Can you work these out from the model? Positions are in its coordinate system, mm. Face numbers are marked on the shaded views. A direction names the side the tool comes from. Round coordinates to 2 decimals unless told otherwise and drop trailing zeros. Loops run counter-clockwise (first coordinate to the right, second up) from the corner with the lowest first, then second, coordinate; pieces in that order, holes last. Notation, with made-up numbers: M 52.25,-30 L 65.25,-30 A38 ccw 65.25,8 Z; hole C 67,17 d7. An arc over 180 degrees is marked long. Return JSON: item names as keys, results as strings.
```python
from build123d import *

# Parameters (mm, degrees)
SKETCH1_W           = 40
SKETCH1_H           = 40
BOSS_EXTRUDE1_DEPTH = 12.7
SKETCH2_R           = 2.67558437
CUT_EXTRUDE1_DEPTH  = 8
CUT_EXTRUDE1_TAPER  = 17.5
FILLET1_R           = 3.175
SKETCH3_W           = 7.62
SKETCH3_H           = 1.27
BOSS_EXTRUDE2_DEPTH = 7.62
SKETCH4_W           = 1.27
SKETCH4_H           = 7.62
BOSS_EXTRUDE3_DEPTH = 7.62
SKETCH5_W           = 1.27
SKETCH5_H           = 7.62
BOSS_EXTRUDE4_DEPTH = 7.62
SKETCH6_W           = 7.62
SKETCH6_H           = 1.27
BOSS_EXTRUDE5_DEPTH = 7.62
SKETCH7_R           = 1.6256
CUT_EXTRUDE2_DEPTH  = 7.62


with BuildPart() as part:
    # Sketch1 → Boss-Extrude1 (new body)
    with BuildSketch(Plane.XY):
        with Locations((-32.473746891, -5.437780853)):
            Rectangle(SKETCH1_W, SKETCH1_H)
    extrude(amount=BOSS_EXTRUDE1_DEPTH)

    # Sketch2 → Cut-Extrude1 (cut)
    with BuildSketch(Plane.XY.offset(12.7)):
        with Locations((-45.973746891, 8.062219147)):
            Circle(SKETCH2_R)
        with Locations((-36.973746891, 8.062219147)):
            Circle(SKETCH2_R)
        with Locations((-27.973746891, 8.062219147)):
            Circle(SKETCH2_R)
        with Locations((-18.973746891, 8.062219147)):
            Circle(SKETCH2_R)
        with Locations((-45.973746891, -0.937780853)):
            Circle(SKETCH2_R)
        with Locations((-36.973746891, -0.937780853)):
            Circle(SKETCH2_R)
        with Locations((-27.973746891, -0.937780853)):
            Circle(SKETCH2_R)
        with Locations((-18.973746891, -0.937780853)):
            Circle(SKETCH2_R)
        with Locations((-45.973746891, -9.937780853)):
            Circle(SKETCH2_R)
        with Locations((-36.973746891, -9.937780853)):
            Circle(SKETCH2_R)
        with Locations((-27.973746891, -9.937780853)):
            Circle(SKETCH2_R)
        with Locations((-18.973746891, -9.937780853)):
            Circle(SKETCH2_R)
        with Locations((-45.973746891, -18.937780853)):
            Circle(SKETCH2_R)
        with Locations((-36.973746891, -18.937780853)):
            Circle(SKETCH2_R)
        with Locations((-27.973746891, -18.937780853)):
            Circle(SKETCH2_R)
        with Locations((-18.973746891, -18.937780853)):
            Circle(SKETCH2_R)
    extrude(amount=-CUT_EXTRUDE1_DEPTH, taper=CUT_EXTRUDE1_TAPER, mode=Mode.SUBTRACT)

    # Fillet1
    fillet1_edges = [part.edges().sort_by_distance(p)[0] for p in [
        (-52.473746891, 14.562219147, 6.35),
        (-12.473746891, 14.562219147, 6.35),
        (-12.473746891, -25.437780853, 6.35),
        (-52.473746891, -25.437780853, 6.35),
    ]]
    fillet(fillet1_edges, radius=FILLET1_R)

    # Sketch3 → Boss-Extrude2 (add)
    with BuildSketch(Plane(origin=(0, 14.562219147, 0), x_dir=(1, 0, 0), z_dir=(0, 1, 0))):
        with Locations((-32.473706891, -0.635)):
            Rectangle(SKETCH3_W, SKETCH3_H)
    extrude(amount=BOSS_EXTRUDE2_DEPTH)

    # Sketch4 → Boss-Extrude3 (add)
    with BuildSketch(Plane(origin=(-12.473746891, 0, 0), x_dir=(0, 0, -1), z_dir=(1, 0, 0))):
        with Locations((-0.635, -5.437820853)):
            Rectangle(SKETCH4_W, SKETCH4_H)
    extrude(amount=BOSS_EXTRUDE3_DEPTH)

    # Sketch5 → Boss-Extrude4 (add)
    with BuildSketch(Plane.ZY.offset(52.473746891)):
        with Locations((0.635, -5.437740853)):
            Rectangle(SKETCH5_W, SKETCH5_H)
    extrude(amount=BOSS_EXTRUDE4_DEPTH)

    # Sketch6 → Boss-Extrude5 (add)
    with BuildSketch(Plane.XZ.offset(25.437780853)):
        with Locations((-32.473786891, 0.635)):
            Rectangle(SKETCH6_W, SKETCH6_H)
    extrude(amount=BOSS_EXTRUDE5_DEPTH)

    # Sketch7 → Cut-Extrude2 (cut)
    with BuildSketch(Plane.XY.offset(1.27)):
        with Locations((-32.473786891, -29.247780853)):
            Circle(SKETCH7_R)
        with Locations((-56.283746891, -5.437740853)):
            Circle(SKETCH7_R)
        with Locations((-8.663746891, -5.437820853)):
            Circle(SKETCH7_R)
        with Locations((-32.473706891, 18.372219147)):
            Circle(SKETCH7_R)
    extrude(amount=-CUT_EXTRUDE2_DEPTH, mode=Mode.SUBTRACT)


solid = part.part
```
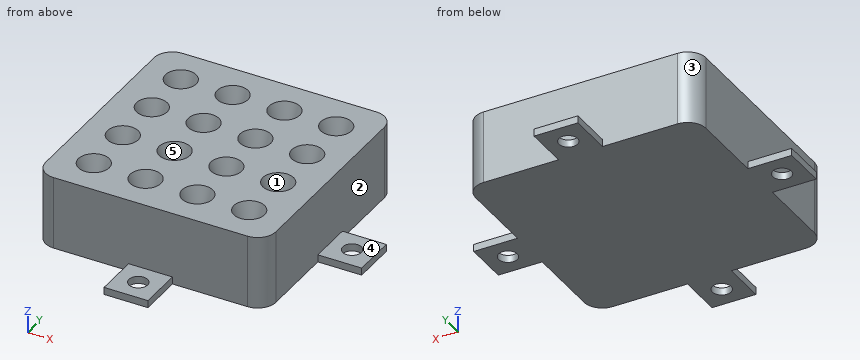
Q1. Suppose I cut it at A-A, the plane z = 10.5. State how many separate pieces and enclosed holes the cut face has, plus the area to 3 significant figures.
Results:
{"separate pieces": "1", "enclosed holes": "16", "area": "1,390 mm2"}
Q2. On a 3-axis mill with a long thin cutter (end or side, diameter ignored), from which of +Z, -Z, +X, -X, +Y, -Y can I reach the whole of each face in a straight line? I mean the marked faces 4 and 5. Say none if no direction works.
Results:
{"face 4": "+Z, +X, +Y, -Y", "face 5": "+Z"}
Q3. If I drill on line 1 along X through (y, z) = (-20.5, 11.75); line 2 along X through (y, z) = (-8.5, 10.5); line 3 along Y through (x, z) = (-18, 8), over which ranges is the centre line in solid material (lowest first)?
Results:
{"line 1": "x = -52.47 to -47.76, -44.18 to -38.76, -35.18 to -29.76, -26.18 to -20.76, -17.18 to -12.47", "line 2": "x = -52.47 to -47.34, -44.61 to -38.34, -35.61 to -29.34, -26.61 to -20.34, -17.61 to -12.47", "line 3": "y = -25.44 to -19.63, -18.25 to -10.63, -9.25 to -1.63, -0.25 to 7.37, 8.75 to 14.56"}
Q4. Thinking about a two-plate mould opening in Y: for the marked faces 1, 2 and 3, which applies, pulls with the +Y half, pulls with the -Y half, needs draft (parallel to the pull), parting line crosses it, or undercut?
Results:
{"face 1": "undercut", "face 2": "needs draft", "face 3": "pulls with the +Y half"}
Q5. Suppose I cut it at D-D, the plane y = 3. Please give me the cut outline in (x, z).
Results:
{"outline": "M -52.47,0 L -12.47,0 L -12.47,12.7 L -52.47,12.7 Z"}
Q6. Suppose I cut it at C-C, the plane x = -11. Please give me the cut outline in (y, z).
Results:
{"outline": "M -9.25,0 L -1.63,0 L -1.63,1.27 L -9.25,1.27 Z"}
Q7. Suppose I cut it at B-B, the plane x = -56. Please give me the cut outline in (y, z).
Results:
{"outline": "M -9.25,0 L -7.04,0 L -7.04,1.27 L -9.25,1.27 Z; M -3.84,0 L -1.63,0 L -1.63,1.27 L -3.84,1.27 Z"}
Q8. I'm going to push flat-ended pins straight in: pin 1 Ø1.5 at (x, z) = (-27.5, 6) entering from -Y; pin 2 Ø4 at (y, z) = (-8, 3.5) entering from -X; pin 3 Ø4 at (y, z) = (-13, 4.5) entering from +X. Where does each tip first touch, or does it pass through?
Results:
{"pin 1": "stops at y = -25.44", "pin 2": "stops at x = -52.47", "pin 3": "stops at x = -12.47"}
